from build123d import *

# Parameters (mm, degrees)
BOSS_EXTRUDE1_DEPTH      = 1100
BOSS_EXTRUDE1_DEPTH_BACK = 300
SKETCH3_R                = 7.5
BOSS_EXTRUDE2_DEPTH      = 800
SKETCH5_R                = 7.5
CUT_EXTRUDE2_DEPTH       = 1519.191769837
SKETCH9_W                = 580
SKETCH9_H                = 60
SKETCH9_W_2              = 60
CUT_EXTRUDE5_DEPTH       = 1486.505638628
SKETCH6_W                = 25
SKETCH6_H                = 32
BOSS_EXTRUDE3_DEPTH      = 37.5
SKETCH7_W                = 16
SKETCH7_H                = 32.5
CUT_EXTRUDE3_DEPTH       = 1507.17537239
SKETCH8_W                = 16
SKETCH8_H                = 64
CUT_EXTRUDE4_DEPTH       = 24
SKETCH10_R               = 2.5908
CUT_EXTRUDE6_DEPTH       = 20


with BuildPart() as part:
    # Sketch2 → Boss-Extrude1 (new, two sides: drawn at the far end of the back side and taken through both)
    with BuildSketch(Plane.XY.offset(-BOSS_EXTRUDE1_DEPTH_BACK)):
        Polygon((0, 0), (0, 81.865758383), (-142.5, 30), (-1042.5, 30), (-1042.5, 0), align=None)
    extrude(amount=BOSS_EXTRUDE1_DEPTH + BOSS_EXTRUDE1_DEPTH_BACK)

    # Sketch3 → Boss-Extrude2 (add)
    # profile 1 of 2: a face of its own
    with BuildSketch(Plane.XY):
        with BuildLine():
            Line((-47.5, 0), (-47.5, -50))
            ThreePointArc((-47.5, -50), (-50.428932188, -57.071067812), (-57.5, -60))
            Line((-57.5, -60), (-512.5, -60))
            ThreePointArc((-512.5, -60), (-519.571067812, -57.071067812), (-522.5, -50))
            Line((-522.5, -50), (-522.5, 0))
            Line((-522.5, 0), (-47.5, 0))
        make_face()
        with BuildLine():
            Line((-510, -42.5), (-60, -42.5))
            ThreePointArc((-60, -42.5), (-52.5, -50), (-60, -57.5))
            Line((-60, -57.5), (-510, -57.5))
            ThreePointArc((-510, -57.5), (-517.5, -50), (-510, -42.5))
        make_face(mode=Mode.SUBTRACT)
    # profile 2 of 2: a face of its own
    with BuildSketch(Plane.XY):
        with BuildLine():
            Line((-1022.5, 0), (-1022.5, -50))
            ThreePointArc((-1022.5, -50), (-1019.571067812, -57.071067812), (-1012.5, -60))
            Line((-1012.5, -60), (-1007.5, -60))
            ThreePointArc((-1007.5, -60), (-1000.428932188, -57.071067812), (-997.5, -50))
            Line((-997.5, -50), (-997.5, 0))
            Line((-997.5, 0), (-1022.5, 0))
        make_face()
        with Locations((-1010, -50)):
            Circle(SKETCH3_R, mode=Mode.SUBTRACT)
    extrude(amount=BOSS_EXTRUDE2_DEPTH)

    # Sketch5 → Cut-Extrude2 (cut, through all)
    with BuildSketch(Plane(origin=(0, 30, 0), x_dir=(1, 0, 0), z_dir=(0, 1, 0))):
        with Locations(Location((-892.5, 0, 0), (0, 0, 180))):
            Circle(SKETCH5_R)
    extrude(amount=-CUT_EXTRUDE2_DEPTH, mode=Mode.SUBTRACT)

    # Sketch9 → Cut-Extrude5 (cut, through all)
    with BuildSketch(Plane(origin=(-47.5, 0, 0), x_dir=(0, 0, -1), z_dir=(1, 0, 0))):
        with Locations((-400, -30)):
            Rectangle(SKETCH9_W, SKETCH9_H)
        Polygon((-740, -50), (-740, -60), (-800, -60), (-800, -50), (-800, 0), (-740, 0), align=None)
        with Locations((-30, -30)):
            Rectangle(SKETCH9_W_2, SKETCH9_H)
    extrude(amount=-CUT_EXTRUDE5_DEPTH, mode=Mode.SUBTRACT)

    # Sketch6 → Boss-Extrude3 (add)
    with BuildSketch(Plane.XZ):
        with Locations((-892.5, 0)):
            Rectangle(SKETCH6_W, SKETCH6_H)
    extrude(amount=BOSS_EXTRUDE3_DEPTH)

    # Sketch7 → Cut-Extrude3 (cut, through all)
    with BuildSketch(Plane.XY.offset(16)):
        with Locations((-892.5, -16.25)):
            Rectangle(SKETCH7_W, SKETCH7_H)
    extrude(amount=-CUT_EXTRUDE3_DEPTH, mode=Mode.SUBTRACT)

    # Sketch8 → Cut-Extrude4 (cut)
    with BuildSketch(Plane.XZ):
        with Locations((-892.5, 0)):
            Rectangle(SKETCH8_W, SKETCH8_H)
    extrude(amount=-CUT_EXTRUDE4_DEPTH, mode=Mode.SUBTRACT)

    # Sketch10 → Cut-Extrude6 (cut)
    with BuildSketch(Plane(origin=(0, 30, 0), x_dir=(1, 0, 0), z_dir=(0, 1, 0))):
        with Locations(Location((-892.5, -1075, 0), (0, 0, 180))):
            Circle(SKETCH10_R)
        with Locations(Location((-592.5, -1075, 0), (0, 0, 180))):
            Circle(SKETCH10_R)
        with Locations(Location((-292.5, -1075, 0), (0, 0, 180))):
            Circle(SKETCH10_R)
        with Locations(Location((-905.2, -420.95, 0), (0, 0, 180))):
            Circle(SKETCH10_R)
        with Locations(Location((-879.8, -420.95, 0), (0, 0, 180))):
            Circle(SKETCH10_R)
        with Locations(Location((-605.2, -420.95, 0), (0, 0, 180))):
            Circle(SKETCH10_R)
        with Locations(Location((-579.8, -420.95, 0), (0, 0, 180))):
            Circle(SKETCH10_R)
        with Locations(Location((-305.2, -420.95, 0), (0, 0, 180))):
            Circle(SKETCH10_R)
        with Locations(Location((-279.8, -420.95, 0), (0, 0, 180))):
            Circle(SKETCH10_R)
    extrude(amount=-CUT_EXTRUDE6_DEPTH, mode=Mode.SUBTRACT)


solid = part.part
Model file for the job. Use its own axes, mm. A direction names the side the tool comes from. Round coordinates to 2 decimals unless told otherwise and drop trailing zeros. Loops run counter-clockwise (first coordinate to the right, second up) from the corner with the lowest first, then second, coordinate; pieces in that order, holes last. Notation, with made-up numbers: (36.5, 44.25) - (78.5, 44.25) arc R26 cw to (78.5, 83.25) - close; hole circle Ø9 at (-25.75, 36.5). An arc over 180 degrees is marked (long way). Write each question's results on one line, items separated by ' | '.
(1) Saw through at D-D, the plane x = -121.5. List the corners of the cut face in (y, z).
Answer below:
outline: (-60, 60) - (-57.5, 60) - (-57.5, 110) - (-60, 110) - close; (-60, 690) - (-57.5, 690) - (-57.5, 740) - (-60, 740) - close; (-42.5, 60) - (0, 60) - (0, -300) - (37.64, -300) - (37.64, 1100) - (0, 1100) - (0, 740) - (-42.5, 740) - (-42.5, 690) - (0, 690) - (0, 110) - (-42.5, 110) - close
(2) 3-axis set-ups, long thin cutter, end or side, ignore diameter. For faces 1 (the flat face through (-288, -42.5, 715)), 2 (the flat face through (-47.5, -25, 715)), 3 (the flat face through (-997.5, -25, 715)), 4 (the flat face through (-282, -17, 690)): which of +Z, -Z, +X, -X, +Y, -Y reach the whole face in a straight line?
Answer below:
face 1: +Z, -Z | face 2: +Z, -Z, +X, -Y | face 3: +Z, -Z, -Y | face 4: +X, -X, -Y
(3) Pin check, flat tips, straight feed: pin 1 (3 mm diameter, centred on x = -292.5, z = 1075, fed in from -Y); pin 2 (12 mm diameter, centred on y = -28, z = 57.5, fed in from -X); pin 3 (6 mm diameter, centred on x = -241, y = -14.5, fed in from -Z); pin 4 (7.5 mm diameter, centred on x = -889, y = -14, fed in from -Z). Stop position of each tip, or through.
Answer below:
pin 1: stops at y = 0 | pin 2: stops at x = -1022.5 | pin 3: stops at z = 60 | pin 4: passes through
(4) Saw through at C-C, the plane x = -759. List the corners of the cut face in (y, z), then the cut area to 3 significant figures.
Answer below:
outline: (0, -300) - (30, -300) - (30, 1100) - (0, 1100) - close | area: 42,000 mm^2
(5) Saw through at B-B, the plane z = 200.5. List the corners of the cut face in (x, y), then the cut area to 3 significant figures.
Answer below:
outline: (-1042.5, 0) - (0, 0) - (0, 81.87) - (-142.5, 30) - (-1042.5, 30) - close | area: 35,000 mm^2
(6) Saw through at A-A, the plane x = -378. List the corners of the cut face in (y, z).
Answer below:
outline: (-60, 60) - (-57.5, 60) - (-57.5, 110) - (-60, 110) - close; (-60, 690) - (-57.5, 690) - (-57.5, 740) - (-60, 740) - close; (-42.5, 60) - (0, 60) - (0, -300) - (30, -300) - (30, 1100) - (0, 1100) - (0, 740) - (-42.5, 740) - (-42.5, 690) - (0, 690) - (0, 110) - (-42.5, 110) - close
(7) Wall check: L1, parallel to X at y = 22.5, z = 1075; L2, parallel to X at y = -50, z = 702.5; L3, parallel to Z at x = -579.8, y = 24. Give the ranges that are in metal, low to high.
Answer below:
L1: x = -1042.5 to -895.09, -889.91 to -595.09, -589.91 to -295.09, -289.91 to 0 | L2: x = -1022.5 to -1017.5, -1002.5 to -997.5, -522.5 to -517.5, -52.5 to -47.5 | L3: z = -300 to 418.36, 423.54 to 1100
(8) Mould opens along Z. For faces 5 (the flat face through (-900.5, 2, 0)), 6 (the flat face through (-288, -42.5, 85)), 7 (the flat face through (-529, 14, -300)) say: released by +Z, released by -Z, zero draft, split by the parting line, or undercut.
Answer below:
face 5: undercut | face 6: zero draft | face 7: released by -Z
